from build123d import *

# Parameters (mm, degrees)
SKETCH1_R           = 32.5
SKETCH1_R_2         = 27.5
BOSS_EXTRUDE1_DEPTH = 7.5
FILLET1_R           = 2
SKETCH3_R           = 4.2
BOSS_EXTRUDE2_DEPTH = 18.85
SKETCH4_R           = 27.5
SKETCH4_R_2         = 22.5
BOSS_EXTRUDE3_DEPTH = 6
SKETCH5_R           = 22.5
SKETCH5_R_2         = 4.2
BOSS_EXTRUDE4_DEPTH = 2.5
CUT_EXTRUDE1_START  = -12.35
SKETCH7_RX          = 5.5
SKETCH7_RY          = 3.5
CUT_EXTRUDE1_DEPTH  = 20.85
CIRPATTERN1_COUNT   = 8


with BuildPart() as part:
    # Sketch1 → Boss-Extrude1 (new body, symmetric)
    with BuildSketch(Plane.XY):
        Circle(SKETCH1_R)
        Circle(SKETCH1_R_2, mode=Mode.SUBTRACT)
    extrude(amount=BOSS_EXTRUDE1_DEPTH, both=True)

    # Fillet1
    fillet1_edges = [part.edges().sort_by_distance(p)[0] for p in [
        (-32.5, 0, -7.5),
        (-32.5, 0, 7.5),
    ]]
    fillet(fillet1_edges, radius=FILLET1_R)

    # Sketch4 → Boss-Extrude3 (add, symmetric)
    with BuildSketch(Plane.XY):
        Circle(SKETCH4_R)
        Circle(SKETCH4_R_2, mode=Mode.SUBTRACT)
    extrude(amount=BOSS_EXTRUDE3_DEPTH, both=True)



with BuildPart() as body_2:
    # Sketch3 → Boss-Extrude2 (new body)
    with BuildSketch(Plane.XY.offset(7.5)):
        Circle(SKETCH3_R)
        with BuildLine():
            Line((-2, 1.813835715), (-2, -1.813835715))
            ThreePointArc((-2, -1.813835715), (0, -2.7), (2, -1.813835715))
            Line((2, -1.813835715), (2, 1.813835715))
            ThreePointArc((2, 1.813835715), (0, 2.7), (-2, 1.813835715))
        make_face(mode=Mode.SUBTRACT)
    extrude(amount=-BOSS_EXTRUDE2_DEPTH)


with BuildPart() as part_1:
    add(part.part)

    add(body_2.part)  # Boss-Extrude4 merges body 2
    # Sketch5 → Boss-Extrude4 (add, symmetric)
    with BuildSketch(Plane.XY):
        Circle(SKETCH5_R)
        Circle(SKETCH5_R_2, mode=Mode.SUBTRACT)
    extrude(amount=BOSS_EXTRUDE4_DEPTH, both=True)

    # Sketch7 → Cut-Extrude1 (cut)
    with BuildSketch(Plane.XY.offset(CUT_EXTRUDE1_START)):
        with Locations(Location((0, 14), (0, 0, 90))):
            Ellipse(SKETCH7_RX, SKETCH7_RY)
    cut_extrude1 = extrude(amount=CUT_EXTRUDE1_DEPTH, mode=Mode.SUBTRACT)

    # CirPattern1: Cut-Extrude1 ×8 about axis
    cirpattern1_axis = Axis((0, 0, 6), (0, 0, -1))
    for i in range(1, CIRPATTERN1_COUNT):
        add(cut_extrude1.rotate(cirpattern1_axis, i * 360 / CIRPATTERN1_COUNT), mode=Mode.SUBTRACT)


solid = part_1.part
Read the model definition and answer for the solid it produces. Units are mm, in the model's axes. A direction names the side the tool comes from. Give positions to 0.01 mm unless a question says otherwise; leave off trailing zeros. Write each loop counter-clockwise with the first axis right and the second up, starting at its lowest first coordinate (ties: lowest second). Pieces come first, ordered by that corner, then holes. Notation, with made-up numbers: (-30, -34) - (22, -34) arc R22 ccw to (22, -1) - close; hole circle Ø8 at (70.25, 4). An arc over 180 degrees is marked (long way). Return JSON: item names as keys, results as strings.
Q1. For faces 4 (the face through (-23, 0, -6)), 5 (the face through (4.006, 1.262, 5.035)), 6 (the face through (0, 2.7, -1.8)), determine the directions among +Z, -Z, +X, -X, +Y, -Y from which every point of the face is accessible in a straight line to the end or side of a thin tool.
Reply:
{"face 4": "-Z", "face 5": "+Z", "face 6": "+Z, -Z"}
Q2. A cutting plane is placed at A-A, the plane z = -9. Determine the outline of the cut face in (x, y), and give its area (3 significant figures).
Reply:
{"outline": "circle Ø8.4 at (0, 0); hole (-2, -1.81) arc R2.7 ccw to (2, -1.81) - (2, 1.81) arc R2.7 ccw to (-2, 1.81) - close", "area": "36.0 mm²"}
Q3. A cutting plane is placed at B-B, the plane y = 0. Count the separate pieces of the cut face and the enclosed holes in it, and give its area (3 significant figures).
Reply:
{"separate pieces": "4", "enclosed holes": "0", "area": "423 mm²"}
Q4. For a pull along Y with two mould halves and no side action, classify faces 1 (the face through (-5.961, -26.846, 6.74)), 2 (the face through (-4.7, 27.3, -7.5)), 3 (the face through (31, 9.76, 0.08)) as released by +Y, released by -Y, zero draft, split by the parting line, or undercut.
Reply:
{"face 1": "undercut", "face 2": "zero draft", "face 3": "split by the parting line"}
Q5. Consider line 1 along X through (y, z) = (1, 5.75); line 2 along X through (y, z) = (-6, 2) (3 decimals); line 3 along Z through (x, y) = (-20.5, 21). Determine where each line is inside the solid, lowest interval first. Write a range as [from, to].
Reply:
{"line 1": "[-32.47, -22.48], [-4.08, -2], [2, 4.08], [22.48, 32.47]", "line 2": "[-31.941, -10.475], [-6.021, 6.021], [10.475, 31.941]", "line 3": "[-7.5, 7.5]"}
Q6. Given P1, Ø10, axis at x = 9.5, z = -9, coming from the +Y side; P2, Ø4, axis at x = 26, y = -2.5, coming from the -Z side; P3, Ø3, axis at x = 10.5, y = 2, coming from the +Z side, each flat-ended and moving along its own axis, determine where each tip first touches the part or whether it passes through.
Reply:
{"P1": "y = 31.98", "P2": "z = -7.5", "P3": "z = 2.5"}
